from build123d import *

# Parameters (mm, degrees)
SKETCH1_R           = 3.175
SKETCH1_W           = 3.2
SKETCH1_H           = 3.2
BOSS_EXTRUDE1_DEPTH = 4.7752
FILLET1_R           = 0.43


with BuildPart() as part:
    # Sketch1 → Boss-Extrude1 (new body)
    with BuildSketch(Plane.XY):
        Circle(SKETCH1_R)
        Rectangle(SKETCH1_W, SKETCH1_H, mode=Mode.SUBTRACT)
    extrude(amount=BOSS_EXTRUDE1_DEPTH)

    # Fillet1
    fillet1_edges = [part.edges().sort_by_distance(p)[0] for p in [
        (1.6, -1.6, 2.3876),
        (1.6, 1.6, 2.3876),
        (-1.6, 1.6, 2.3876),
        (-1.6, -1.6, 2.3876),
    ]]
    fillet(fillet1_edges, radius=FILLET1_R)


solid = part.part
Check sheet for the modelled part. Datum: model origin and axes. Units: mm. A direction names the side the tool comes from. Give positions to 0.01 mm unless a question says otherwise; leave off trailing zeros. Loops run counter-clockwise (first coordinate to the right, second up) from the corner with the lowest first, then second, coordinate; pieces in that order, holes last. Notation, with made-up numbers: M -5,66.5 L 25,66.5 A20 ccw 25,99.5 Z; hole C -5.5,-13 d9. An arc over 180 degrees is marked long. Return JSON: item names as keys, results as strings. Group by question number.
1. Thickness scan on L1, parallel to Y at x = 0.5, z = 3.2; L2, parallel to Y at x = -1.25, z = 3.65; L3, parallel to X at y = 0.25, z = 2.55. Record the ranges inside material, lowest first.
2. Cross-section at C-C on z = 1.45. Record the boundary of the cut face in (x, y) (3 decimals).
3. Mould release check, pull along Y, two halves, no side actions. Record for faces 3 (the flat face through (0, -2, 0)), 4 (the cylindrical face through (-0.69, -3.1, 2.35)), 5 (the flat face through (-1.6, 0, 2)): released by +Y, released by -Y, zero draft, split by the parting line, or undercut.
4. Cross-section at A-A on y = 0. Record the boundary of the cut face in (x, z) (3 decimals), plus the area to 3 significant figures.
5. Go/stop test with a flat-tipped pin: pin 1 (0.7 mm diameter, centred on x = -0.5, z = 2.5, fed in from -Y). Record where the tip stops, or that it passes through.
6. Cross-section at D-D on y = 2.5. Record the boundary of the cut face in (x, z).
7. Tool access check on faces 1 (the flat face through (0, -2, 4.775)), 2 (the flat face through (0, 1.6, 2)). Record the directions out of +Z, -Z, +X, -X, +Y, -Y that give a thin tool (end or side, any length) a straight path to the whole face; none if there is none.
Return value:
{
 "1": {"L1": "-3.14 to -1.6, 1.6 to 3.14", "L2": "-2.92 to -1.59, 1.59 to 2.92", "L3": "-3.17 to -1.6, 1.6 to 3.17"},
 "2": {"outline": "C 0,0 d6.35; hole M -1.6,-1.17 A0.43 ccw -1.17,-1.6 L 1.17,-1.6 A0.43 ccw 1.6,-1.17 L 1.6,1.17 A0.43 ccw 1.17,1.6 L -1.17,1.6 A0.43 ccw -1.6,1.17 Z"},
 "3": {"face 3": "zero draft", "face 4": "split by the parting line", "face 5": "undercut"},
 "4": {"outline": "M -3.175,0 L -1.6,0 L -1.6,4.775 L -3.175,4.775 Z; M 1.6,0 L 3.175,0 L 3.175,4.775 L 1.6,4.775 Z", "area": "15.0 mm^2"},
 "5": {"pin 1": "y = -3.17"},
 "6": {"outline": "M -1.96,0 L 1.96,0 L 1.96,4.78 L -1.96,4.78 Z"},
 "7": {"face 1": "+Z, +X, -X, +Y, -Y", "face 2": "+Z, -Z"}
}
